Here's the drawing with two shaded views (mm, measured from the low corner). I have some questions. A direction names the side the tool comes from. Coordinates: 2 decimals unless noted, no trailing zeros. Write each loop counter-clockwise with the first axis right and the second up, starting at its lowest first coordinate (ties: lowest second). Pieces come first, ordered by that corner, then holes. Notation, with made-up numbers: M 51,17.25 L 105,17.25 A13 cw 105,27.25 Z; hole C -5.5,26.5 d11. An arc over 180 degrees is marked long. Answer as CSV lines item,"result". Start each with the question number.
Item 1: I'm going to push flat-ended pins straight in: P1, Ø1.5, axis at x = 1.5, y = 1, coming from the +Z side; P2, Ø3, axis at x = 3, z = 3.5, coming from the -Y side; P3, Ø1.4, axis at y = 1.5, z = 1, coming from the +X side; P4, Ø1, axis at y = 3, z = 8.5, coming from the -X side. Where does each tip first touch, or does it pass through?
Item 2: Suppose I cut it at C-C, the plane y = 1.45. Write out the boundary of the cut face in (x, z).
Item 3: On a 3-axis mill with a long thin cutter (end or side, diameter ignored), from which of +Z, -Z, +X, -X, +Y, -Y can I reach the whole of each face in a straight line? I mean the marked faces 4 and 5. Say none if no direction works.
Item 4: Suppose I cut it at B-B, the plane z = 4.5. Write out the boundary of the cut face in (x, y), and give its area (3 significant figures).
Item 5: Suppose I cut it at A-A, the plane x = 3.2. Write out the boundary of the cut face in (y, z).
Item 6: We'd pull the mould along Z, two halves only. Please class the marked faces 1, 2 and 3: +Z half, -Z half, draft (parallel to the pull), parting line (faces both ways), or undercut.
Item 7: If I drill on line 1 along X through (y, z) = (3.75, 4.5); line 2 along Z through (x, y) = (4, 0.6); line 3 along X through (y, z) = (3.55, 5.5), over which ranges is the centre line in solid material (lowest first)? Write a range as [from, to].
Item 8: Suppose I cut it at D-D, the plane y = 3.6. Write out the boundary of the cut face in (x, z).
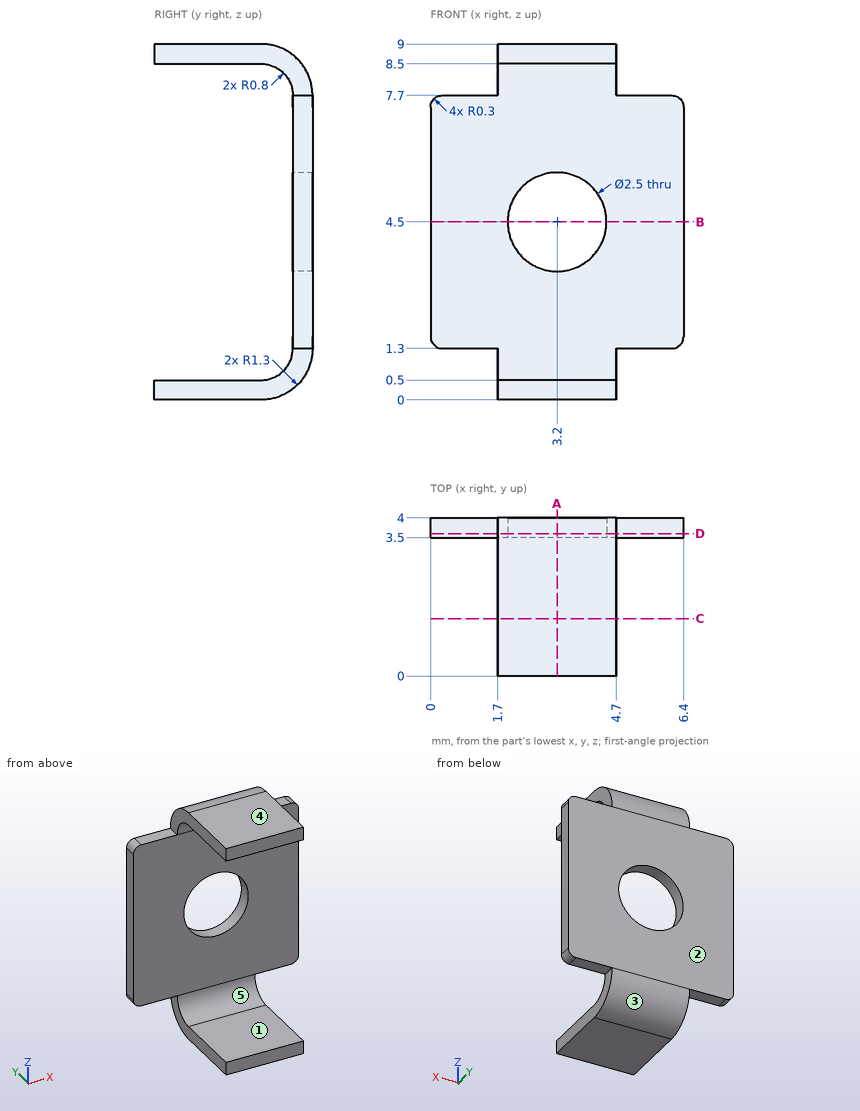
Ans:
1,P1,"stops at z = 9"
1,P2,"stops at y = 3.5"
1,P3,"stops at x = 4.7"
1,P4,"stops at x = 1.7"
2,outline,"M 1.7,0 L 4.7,0 L 4.7,0.5 L 1.7,0.5 Z; M 1.7,8.5 L 4.7,8.5 L 4.7,9 L 1.7,9 Z"
3,face 4,"+Z, +X, -X, +Y, -Y"
3,face 5,"+X, -X, -Y"
4,outline,"M 0,3.5 L 1.95,3.5 L 1.95,4 L 0,4 Z; M 4.45,3.5 L 6.4,3.5 L 6.4,4 L 4.45,4 Z"
4,area,"1.95 mm^2"
5,outline,"M 0,0 L 2.7,0 A1.3 ccw 4,1.3 L 4,3.25 L 3.5,3.25 L 3.5,1.3 A0.8 cw 2.7,0.5 L 0,0.5 Z; M 0,8.5 L 2.7,8.5 A0.8 cw 3.5,7.7 L 3.5,5.75 L 4,5.75 L 4,7.7 A1.3 ccw 2.7,9 L 0,9 Z"
6,face 1,"undercut"
6,face 2,"draft"
6,face 3,"-Z half"
7,line 1,"x = [0, 1.95], [4.45, 6.4]"
7,line 2,"z = [0, 0.5], [8.5, 9]"
7,line 3,"x = [0, 2.45], [3.95, 6.4]"
8,outline,"M 0,1.6 A0.3 ccw 0.3,1.3 L 1.7,1.3 L 1.7,0.36 L 4.7,0.36 L 4.7,1.3 L 6.1,1.3 A0.3 ccw 6.4,1.6 L 6.4,7.4 A0.3 ccw 6.1,7.7 L 4.7,7.7 L 4.7,8.64 L 1.7,8.64 L 1.7,7.7 L 0.3,7.7 A0.3 ccw 0,7.4 Z; hole C 3.2,4.5 d2.5"
